from build123d import *

# Parameters (mm, degrees)
SKETCH1_W           = 85
SKETCH1_H           = 56
BOSS_EXTRUDE1_DEPTH = 2
SKETCH2_R           = 1.5
CUT_EXTRUDE2_DEPTH  = 2
SKETCH3_W           = 20
SKETCH3_H           = 20
BOSS_EXTRUDE2_DEPTH = 2
SKETCH4_W           = 15
SKETCH4_H           = 15
BOSS_EXTRUDE3_DEPTH = 5
SKETCH5_W           = 3
SKETCH5_H           = 15
BOSS_EXTRUDE4_DEPTH = 15
CUT_EXTRUDE3_DEPTH  = 15
CUT_EXTRUDE4_DEPTH  = 15
SKETCH9_R           = 2.5
CUT_EXTRUDE5_DEPTH  = 15
FILLET1_R           = 4
FILLET2_R           = 0.5
FILLET3_R           = 0.5
CUT_EXTRUDE6_DEPTH  = 15


with BuildPart() as part:
    # Sketch1 → Boss-Extrude1 (new body)
    with BuildSketch(Plane(origin=(0, 0, 0), x_dir=(1, 0, 0), z_dir=(0, 1, 0))):
        Rectangle(SKETCH1_W, SKETCH1_H)
    extrude(amount=BOSS_EXTRUDE1_DEPTH)

    # Sketch2 → Cut-Extrude2 (cut)
    with BuildSketch(Plane(origin=(0, 0, 0), x_dir=(1, 0, 0), z_dir=(0, 1, 0))):
        with Locations(Location((-39, -24.5, 0), (0, 0, 270))):
            Circle(SKETCH2_R)
        with Locations(Location((-39, 24.5, 0), (0, 0, 270))):
            Circle(SKETCH2_R)
        with Locations(Location((19, 24.5, 0), (0, 0, 270))):
            Circle(SKETCH2_R)
        with Locations(Location((19, -24.5, 0), (0, 0, 270))):
            Circle(SKETCH2_R)
    extrude(amount=CUT_EXTRUDE2_DEPTH, mode=Mode.SUBTRACT)

    # Sketch3 → Boss-Extrude2 (add)
    with BuildSketch(Plane(origin=(0, 2, 0), x_dir=(1, 0, 0), z_dir=(0, 1, 0))):
        Rectangle(SKETCH3_W, SKETCH3_H)
    extrude(amount=BOSS_EXTRUDE2_DEPTH)

    # Sketch4 → Boss-Extrude3 (add)
    with BuildSketch(Plane(origin=(0, 4, 0), x_dir=(1, 0, 0), z_dir=(0, 1, 0))):
        Rectangle(SKETCH4_W, SKETCH4_H)
    extrude(amount=BOSS_EXTRUDE3_DEPTH)

    # Sketch5 → Boss-Extrude4 (add)
    with BuildSketch(Plane(origin=(0, 9, 0), x_dir=(1, 0, 0), z_dir=(0, 1, 0))):
        Rectangle(SKETCH5_W, SKETCH5_H)
    extrude(amount=BOSS_EXTRUDE4_DEPTH)

    # Sketch7 → Cut-Extrude3 (cut)
    with BuildSketch(Plane.ZY.offset(1.5)):
        with BuildLine():
            Line((-7.5, 16.5), (-7.5, 24))
            Line((-7.5, 24), (0, 24))
            ThreePointArc((0, 24), (-5.303300859, 21.803300859), (-7.5, 16.5))
        make_face()
    extrude(amount=-CUT_EXTRUDE3_DEPTH, mode=Mode.SUBTRACT)

    # Sketch8 → Cut-Extrude4 (cut)
    with BuildSketch(Plane.ZY.offset(1.5)):
        with BuildLine():
            Line((7.5, 16.5), (7.5, 24))
            Line((7.5, 24), (0, 24))
            ThreePointArc((0, 24), (5.303300859, 21.803300859), (7.5, 16.5))
        make_face()
    extrude(amount=-CUT_EXTRUDE4_DEPTH, mode=Mode.SUBTRACT)

    # Sketch9 → Cut-Extrude5 (cut)
    with BuildSketch(Plane.ZY.offset(1.5)):
        with Locations((0, 16.5)):
            Circle(SKETCH9_R)
    extrude(amount=-CUT_EXTRUDE5_DEPTH, mode=Mode.SUBTRACT)

    # Fillet1
    fillet1_edges = [part.edges().sort_by_distance(p)[0] for p in [
        (10, 3, 10),
        (10, 3, -10),
        (-10, 3, -10),
        (-10, 3, 10),
        (7.5, 6.5, 7.5),
        (7.5, 6.5, -7.5),
        (-7.5, 6.5, -7.5),
        (-7.5, 6.5, 7.5),
    ]]
    fillet(fillet1_edges, radius=FILLET1_R)

    # Fillet2
    fillet2_edges = [part.edges().sort_by_distance(p)[0] for p in [
        (7.5, 4, 0),
        (0, 4, 7.5),
        (-7.5, 4, 0),
        (0, 4, -7.5),
        (10, 4, 0),
        (0, 4, 10),
        (0, 4, -10),
        (-10, 4, 0),
        (8.828427125, 4, -8.828427125),
        (-8.828427125, 4, -8.828427125),
        (-8.828427125, 4, 8.828427125),
        (8.828427125, 4, 8.828427125),
        (6.328427125, 4, 6.328427125),
        (-6.328427125, 4, 6.328427125),
        (-6.328427125, 4, -6.328427125),
        (6.328427125, 4, -6.328427125),
    ]]
    fillet(fillet2_edges, radius=FILLET2_R)

    # Fillet3
    fillet3_edges = [part.edges().sort_by_distance(p)[0] for p in [
        (7.5, 9, 0),
        (-2.5, 9, 7.5),
        (2.5, 9, -7.5),
        (6.328427125, 9, -6.328427125),
        (6.328427125, 9, 6.328427125),
        (-7.5, 9, 0),
        (-6.328427125, 9, -6.328427125),
        (-6.328427125, 9, 6.328427125),
        (-2.5, 9, -7.5),
        (2.5, 9, 7.5),
    ]]
    fillet(fillet3_edges, radius=FILLET3_R)

    # Sketch10 → Cut-Extrude6 (cut)
    with BuildSketch(Plane(origin=(0, 2, 0), x_dir=(1, 0, 0), z_dir=(0, 1, 0))):
        with BuildLine():
            Line((-21, -17.5), (-19, -17.5))
            ThreePointArc((-19, -17.5), (-17.585786438, -16.914213562), (-17, -15.5))
            Line((-17, -15.5), (-17, 15.5))
            ThreePointArc((-17, 15.5), (-17.585786438, 16.914213562), (-19, 17.5))
            Line((-19, 17.5), (-21, 17.5))
            ThreePointArc((-21, 17.5), (-22.414213562, 16.914213562), (-23, 15.5))
            Line((-23, 15.5), (-23, -15.5))
            ThreePointArc((-23, -15.5), (-22.414213562, -16.914213562), (-21, -17.5))
        make_face()
        with BuildLine():
            Line((-35, -15.5), (-35, 15.5))
            ThreePointArc((-35, 15.5), (-34.414213562, 16.914213562), (-33, 17.5))
            Line((-33, 17.5), (-31, 17.5))
            ThreePointArc((-31, 17.5), (-29.585786438, 16.914213562), (-29, 15.5))
            Line((-29, 15.5), (-29, -15.5))
            ThreePointArc((-29, -15.5), (-29.585786438, -16.914213562), (-31, -17.5))
            Line((-31, -17.5), (-33, -17.5))
            ThreePointArc((-33, -17.5), (-34.414213562, -16.914213562), (-35, -15.5))
        make_face()
        with BuildLine():
            Line((33, -17.5), (31, -17.5))
            ThreePointArc((31, -17.5), (29.585786438, -16.914213562), (29, -15.5))
            Line((29, -15.5), (29, 15.5))
            ThreePointArc((29, 15.5), (29.585786438, 16.914213562), (31, 17.5))
            Line((31, 17.5), (33, 17.5))
            ThreePointArc((33, 17.5), (34.414213562, 16.914213562), (35, 15.5))
            Line((35, 15.5), (35, -15.5))
            ThreePointArc((35, -15.5), (34.414213562, -16.914213562), (33, -17.5))
        make_face()
        with BuildLine():
            Line((21, 17.5), (19, 17.5))
            ThreePointArc((19, 17.5), (17.585786438, 16.914213562), (17, 15.5))
            Line((17, 15.5), (17, -15.5))
            ThreePointArc((17, -15.5), (17.585786438, -16.914213562), (19, -17.5))
            Line((19, -17.5), (21, -17.5))
            ThreePointArc((21, -17.5), (22.414213562, -16.914213562), (23, -15.5))
            Line((23, -15.5), (23, 15.5))
            ThreePointArc((23, 15.5), (22.414213562, 16.914213562), (21, 17.5))
        make_face()
    extrude(amount=-CUT_EXTRUDE6_DEPTH, mode=Mode.SUBTRACT)


solid = part.part
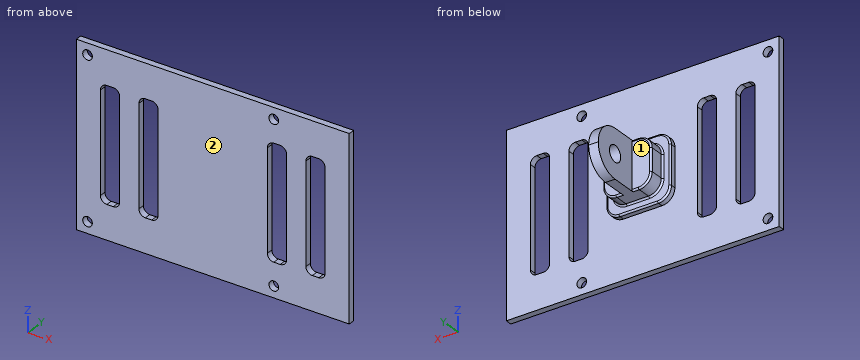
Geometry: final body of the model. Coordinates: model frame, mm. Face numbers are marked on the shaded views. A direction names the side the tool comes from. Give positions to 0.01 mm unless a question says otherwise; leave off trailing zeros. Loops run counter-clockwise (first coordinate to the right, second up) from the corner with the lowest first, then second, coordinate; pieces in that order, holes last. Notation, with made-up numbers: M 56,31 L 100,31 A26 cw 100,45 Z; hole C -28.5,-4.5 d11. An arc over 180 degrees is marked long. Put each result on its own line as item: value. Start each with the question number.
1) Cut plane D-D (y = 11.5). Output: boundary loops of the cut face in (x, z).
2) Cut plane C-C (x = -39). Output: boundary loops of the cut face in (y, z).
3) Contact query for flat-ended pins moving along their axis: pin 1 (0.8 mm diameter, centred on x = 2.5, y = 3, fed in from -Z); pin 2 (5 mm diameter, centred on x = 3, y = 15.5, fed in from +Z); pin 3 (17 mm diameter, centred on x = -5, z = -1.5, fed in from +Y); pin 4 (1 mm diameter, centred on y = 8, z = -6, fed in from +X). Output: stop coordinate, or through.
4) Access query for the marked faces 1 and 2. Directions: +Z, -Z, +X, -X, +Y, -Y. A direction counts if a zero-diameter tool reaches every point of the face in a straight line with its end or side. Return the directions, or none.
5) Cut plane B-B (z = -24.5). Output: boundary loops of the cut face in (x, y), then the cut area to 3 significant figures.
6) Ray query, line 1 along X through (y, z) = (1.45, -24.5); line 2 along Y through (x, z) = (-15, -13.5); line 3 along X through (y, z) = (11, -1.5). Return the intervals inside material, ascending.
7) Cut plane A-A (z = -13). Output: boundary loops of the cut face in (x, y).
Verdict:
1. outline: M -1.5,-7.5 L 1.5,-7.5 L 1.5,7.5 L -1.5,7.5 Z
2. outline: M 0,-28 L 2,-28 L 2,-26 L 0,-26 Z; M 0,-23 L 2,-23 L 2,23 L 0,23 Z; M 0,26 L 2,26 L 2,28 L 0,28 Z
3. pin 1: z = -10
3. pin 2: z = 7.5
3. pin 3: y = 24
3. pin 4: x = 6.96
4. face 1: +Z, -Z, -X, +Y
4. face 2: +Z, -Z, +X, -X, -Y
5. outline: M -42.5,0 L -40.5,0 L -40.5,2 L -42.5,2 Z; M -37.5,0 L 17.5,0 L 17.5,2 L -37.5,2 Z; M 20.5,0 L 42.5,0 L 42.5,2 L 20.5,2 Z
5. area: 158 mm2
6. line 1: -42.5 to -40.5, -37.5 to 17.5, 20.5 to 42.5
6. line 2: 0 to 2
6. line 3: -1.5 to 1.5
7. outline: M -42.5,0 L -35,0 L -35,2 L -42.5,2 Z; M -29,0 L -23,0 L -23,2 L -29,2 Z; M -17,0 L 17,0 L 17,2 L -17,2 Z; M 23,0 L 29,0 L 29,2 L 23,2 Z; M 35,0 L 42.5,0 L 42.5,2 L 35,2 Z
